from build123d import *

# Parameters (mm, degrees)
SKETCH_1_R          = 4
EXTRUDE_1_DEPTH     = 6
SKETCH_2_R          = 6.85
CUT_EXTRUDE_1_DEPTH = 5.2
SKETCH_3_R          = 7.85
CUT_EXTRUDE_2_DEPTH = 1


with BuildPart() as part:
    # 草图1 → 凸台-拉伸1 (new body)
    with BuildSketch(Plane(origin=(0, 0, 0), x_dir=(1, 0, 0), z_dir=(0, 1, 0))):
        Polygon((-65.26232397, 5), (-70.363344484, 10), (-80.363344484, 10), (-85.26232397, 5), (-85.26232397, -5), (-80.363344484, -10), (-70.363344484, -10), (-65.26232397, -5), (72.73767603, -5), (77.636655516, -10), (87.636655516, -10), (92.739759147, -5), (92.739759147, 5), (87.636655516, 10), (77.636655516, 10), (72.73767603, 5), align=None)
        with Locations(Location((-75.363344484, 0, 0), (0, 0, 270))):
            Circle(SKETCH_1_R, mode=Mode.SUBTRACT)
        with Locations(Location((82.636655516, 0, 0), (0, 0, 270))):
            Circle(SKETCH_1_R, mode=Mode.SUBTRACT)
    extrude(amount=EXTRUDE_1_DEPTH)

    # 草图2 → 切除-拉伸1 (cut)
    with BuildSketch(Plane(origin=(0, 6, 0), x_dir=(1, 0, 0), z_dir=(0, 1, 0))):
        with Locations(Location((82.636655516, 0, 0), (0, 0, 270))):
            Circle(SKETCH_2_R)
        with Locations(Location((-75.363344484, 0, 0), (0, 0, 270))):
            Circle(SKETCH_2_R)
    extrude(amount=-CUT_EXTRUDE_1_DEPTH, mode=Mode.SUBTRACT)

    # 草图3 → 切除-拉伸2 (cut)
    with BuildSketch(Plane(origin=(0, 6, 0), x_dir=(1, 0, 0), z_dir=(0, 1, 0))):
        with Locations(Location((82.636655516, 0, 0), (0, 0, 270))):
            Circle(SKETCH_3_R)
        with Locations(Location((-75.363344484, 0, 0), (0, 0, 270))):
            Circle(SKETCH_3_R)
    extrude(amount=-CUT_EXTRUDE_2_DEPTH, mode=Mode.SUBTRACT)


solid = part.part
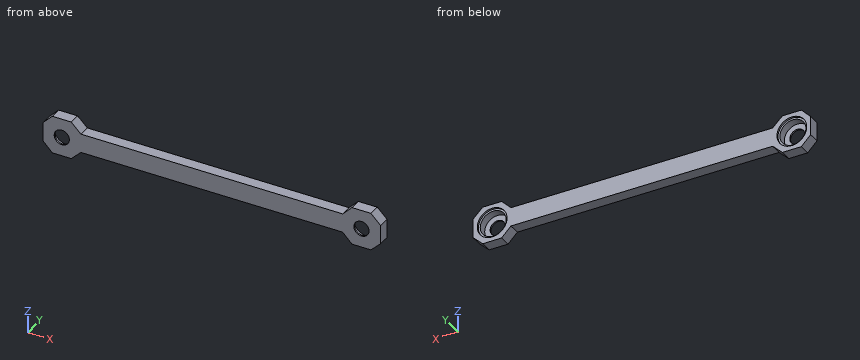
Part model, mm, in its own coordinate system. Coordinates: 2 decimals unless noted, no trailing zeros. Order: outer loops, then holes, each group sorted by start corner. A loop starts at its lowest first (then second) coordinate and runs counter-clockwise, first axis right, second up.
(1) Pin check, flat tips, straight feed: pin 1 Ø8 at (x, z) = (83.5, -2) entering from +Y; pin 2 Ø11 at (x, z) = (84.5, -0.5) entering from +Y; pin 3 Ø3 at (x, y) = (0, 4) entering from -Z; pin 4 Ø7 at (x, z) = (-75.36, 0) entering from +Y. Stop position of each tip, or through.
Check sheet entries:
pin 1: stops at y = 0.8
pin 2: stops at y = 5
pin 3: stops at z = -5
pin 4: passes through
(2) Probe L1, parallel to X at y = 5.65, z = 0; L2, parallel to X at y = 2.45, z = 0; L3, parallel to Z at x = 65, y = 0.75. List the from-to ranges inside material, lowest first.
Check sheet entries:
L1: x = -85.26 to -83.21, -67.51 to 74.79, 90.49 to 92.74
L2: x = -85.26 to -82.21, -68.51 to 75.79, 89.49 to 92.74
L3: z = -5 to 5
(3) Slice it at B-B, the plane x = -37. Write the cut outline in (y, z).
Check sheet entries:
outline: (0, -5) - (6, -5) - (6, 5) - (0, 5) - close
(4) Slice it at A-A, the plane z = 0. Write the cut outline in (x, y).
Check sheet entries:
outline: (-85.26, 0) - (-79.36, 0) - (-79.36, 0.8) - (-82.21, 0.8) - (-82.21, 5) - (-83.21, 5) - (-83.21, 6) - (-85.26, 6) - close; (-71.36, 0) - (78.64, 0) - (78.64, 0.8) - (75.79, 0.8) - (75.79, 5) - (74.79, 5) - (74.79, 6) - (-67.51, 6) - (-67.51, 5) - (-68.51, 5) - (-68.51, 0.8) - (-71.36, 0.8) - close; (86.64, 0) - (92.74, 0) - (92.74, 6) - (90.49, 6) - (90.49, 5) - (89.49, 5) - (89.49, 0.8) - (86.64, 0.8) - close
